```python
from build123d import *

# Parameters (mm, degrees)
SKETCH1_W              = 125
SKETCH1_H              = 12
BOSS_EXTRUDE1_DEPTH    = 72
SKETCH2_W              = 125
SKETCH2_H              = 12
BOSS_EXTRUDE2_DEPTH    = 62
SKETCH3_W              = 12
SKETCH3_H              = 74
BOSS_EXTRUDE3_DEPTH    = 15
SKETCH4_W              = 125
SKETCH4_H              = 12
BOSS_EXTRUDE4_DEPTH    = 12
FILLET1_R              = 10
SKETCH5_W              = 12
SKETCH5_H              = 62
BOSS_EXTRUDE5_DEPTH    = 60
CUT_EXTRUDE4_DEPTH     = 12
FILLET2_R              = 10
F_10_0MM_DOWEL_SLOT1_D = 10
F_10_0MM_DOWEL_SLOT2_D = 10


with BuildPart() as part:
    # Sketch1 → Boss-Extrude1 (new body)
    with BuildSketch(Plane.XY):
        Rectangle(SKETCH1_W, SKETCH1_H)
    extrude(amount=-BOSS_EXTRUDE1_DEPTH)

    # Sketch2 → Boss-Extrude2 (add)
    with BuildSketch(Plane(origin=(0, 6, 0), x_dir=(1, 0, 0), z_dir=(0, 1, 0))):
        with Locations((0, 66)):
            Rectangle(SKETCH2_W, SKETCH2_H)
    extrude(amount=BOSS_EXTRUDE2_DEPTH)

    # Sketch3 → Boss-Extrude3 (add)
    with BuildSketch(Plane(origin=(0, 0, -72), x_dir=(-1, 0, 0), z_dir=(0, 0, -1))):
        with Locations((-16.5, 31)):
            Rectangle(SKETCH3_W, SKETCH3_H)
        with Locations((15.5, 31)):
            Rectangle(SKETCH3_W, SKETCH3_H)
    extrude(amount=BOSS_EXTRUDE3_DEPTH)

    # Sketch4 → Boss-Extrude4 (add)
    with BuildSketch(Plane.XZ.offset(6)):
        with Locations((0, -65.675154964)):
            Rectangle(SKETCH4_W, SKETCH4_H)
    extrude(amount=BOSS_EXTRUDE4_DEPTH)

    # Fillet1
    fillet1_edges = [part.edges().sort_by_distance(p)[0] for p in [
        (-62.5, 68, -66),
        (62.5, 68, -66),
    ]]
    fillet(fillet1_edges, radius=FILLET1_R)

    # Sketch5 → Boss-Extrude5 (add)
    with BuildSketch(Plane.XY.offset(-60)):
        with Locations((-0.169803283, 37)):
            Rectangle(SKETCH5_W, SKETCH5_H)
    extrude(amount=BOSS_EXTRUDE5_DEPTH)

    # Sketch6 → Cut-Extrude4 (cut)
    with BuildSketch(Plane.ZY.offset(6.169803283)):
        Polygon((0, 6), (-60, 40.641016151), (-60, 68), (0, 68), align=None)
    extrude(amount=-CUT_EXTRUDE4_DEPTH, mode=Mode.SUBTRACT)

    # Fillet2
    fillet2_edges = [part.edges().sort_by_distance(p)[0] for p in [
        (-0.169803283, 40.641016151, -60),
    ]]
    fillet(fillet2_edges, radius=FILLET2_R)

    # Ø10.0mm Dowel Slot1 (through all)
    with Locations(Plane.XY.offset(-60)):
        with Locations((42.5, 36), (-42.5, 36)):
            Hole(F_10_0MM_DOWEL_SLOT1_D / 2)

    # Ø10.0mm Dowel Slot2 (through all)
    with Locations(Plane(origin=(0, 6, 0), x_dir=(1, 0, 0), z_dir=(0, 1, 0))):
        with Locations((-47.5, 15), (47.5, 45)):
            Hole(F_10_0MM_DOWEL_SLOT2_D / 2)


solid = part.part
```
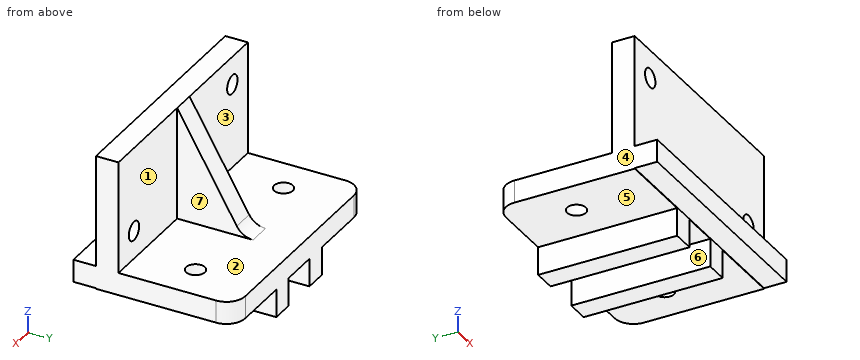
Read the model definition and answer for the solid it produces. Units are mm, in the model's axes. Face numbers are marked on the shaded views. A direction names the side the tool comes from. Give positions to 0.01 mm unless a question says otherwise; leave off trailing zeros. Order: outer loops, then holes, each group sorted by start corner. A loop starts at its lowest first (then second) coordinate and runs counter-clockwise, first axis right, second up.
(1) For a pull along X with two mould halves and no side action, classify the marked faces 4, 5, 6 and 7 as released by +X, released by -X, zero draft, split by the parting line, or undercut.
(2) Straight lines are drawn through the part: L1, parallel to Y at x = 42.5, z = -66.25; L2, parallel to Z at x = -47, y = 2; L3, parallel to Z at x = 47.5, y = -2.5. For each, find the intervals that lie inside material, in ascending order.
(3) Given pin 1 (4.5 mm diameter, centred on y = 33, z = -82.5, fed in from -X); pin 2 (8 mm diameter, centred on x = -24.5, y = 27.5, fed in from +Z); pin 3 (2 mm diameter, centred on y = 46.5, z = -76.5, fed in from +X); pin 4 (9 mm diameter, centred on x = 47.5, z = -45, fed in from -Y), each flat-ended and moving along its own axis, determine where each tip first touches the part or whether it passes through.
(4) Find section D-D (y = 36). Give the vertices of the cut face in (x, z).
(5) For the marked faces 1, 2 and 3, determine the directions among +Z, -Z, +X, -X, +Y, -Y from which every point of the face is accessible in a straight line to the end or side of a thin tool.
(6) Find section C-C (x = 4). Give the vertices of the cut face in (y, z).
(7) Find section A-A (y = 1.5). Give the vertices of the cut face in (x, z), plus the area to 3 significant figures.
(8) Find section B-B (z = -80.5). Give the vertices of the cut face in (x, y), plus the area to 3 significant figures.
Result sheet:
1. face 4: released by -X
1. face 5: zero draft
1. face 6: undercut
1. face 7: released by +X
2. L1: y = -18 to 31, 41 to 68
2. L2: z = -72 to -19.97, -10.03 to 0
2. L3: z = -72 to -50, -40 to 0
3. pin 1: stops at x = -21.5
3. pin 2: stops at z = -60
3. pin 3: stops at x = 22.5
3. pin 4: passes through
4. outline: (-62.5, -72) - (-47.5, -72) - (-47.5, -60) - (-62.5, -60) - close; (-37.5, -72) - (-21.5, -72) - (-21.5, -87) - (-9.5, -87) - (-9.5, -72) - (10.5, -72) - (10.5, -87) - (22.5, -87) - (22.5, -72) - (37.5, -72) - (37.5, -60) - (5.83, -60) - (5.83, -51.96) - (-6.17, -51.96) - (-6.17, -60) - (-37.5, -60) - close; (47.5, -72) - (62.5, -72) - (62.5, -60) - (47.5, -60) - close
5. face 1: +Z, +X, +Y
5. face 2: +Z, +Y
5. face 3: +Z, -X, +Y
6. outline: (-18, -71.68) - (-6, -71.68) - (-6, -72) - (68, -72) - (68, -60) - (46.41, -60) arc R10 cw to (37.75, -55) - (6, 0) - (-6, 0) - (-6, -59.68) - (-18, -59.68) - close
7. outline: (-62.5, -72) - (-21.5, -72) - (-21.5, -87) - (-9.5, -87) - (-9.5, -72) - (10.5, -72) - (10.5, -87) - (22.5, -87) - (22.5, -72) - (62.5, -72) - (62.5, 0) - (-62.5, 0) - close; hole circle Ø10 at (-47.5, -15); hole circle Ø10 at (47.5, -45)
7. area: 9,200 mm2
8. outline: (-21.5, -6) - (-9.5, -6) - (-9.5, 68) - (-21.5, 68) - close; (10.5, -6) - (22.5, -6) - (22.5, 68) - (10.5, 68) - close
8. area: 1,780 mm2
